For this review, take the finished solid that the model builds, in its own axes (mm). Coordinates: 2 decimals unless noted, no trailing zeros. Write each loop counter-clockwise with the first axis right and the second up, starting at its lowest first coordinate (ties: lowest second). Pieces come first, ordered by that corner, then holes. Notation, with made-up numbers: M -35.75,72.25 L 18.25,72.25 A21 cw 18.25,96.25 Z; hole C 27.25,29.25 d4. An arc over 180 degrees is marked long. One line per question, with ' | ' between items.
from build123d import *

# Parameters (mm, degrees)
CROQUIS1_R              = 9
SALIENTE_EXTRUIR1_DEPTH = 25
CROQUIS2_R              = 1.5
CORTAR_EXTRUIR1_DEPTH   = 25


with BuildPart() as part:
    # Croquis1 → Saliente-Extruir1 (new body)
    with BuildSketch(Plane.XY):
        Polygon((-22.5, 5), (-12.5, 15), (12.5, 15), (22.5, 5), (22.5, -15), (-22.5, -15), align=None)
        Circle(CROQUIS1_R, mode=Mode.SUBTRACT)
    extrude(amount=SALIENTE_EXTRUIR1_DEPTH)

    # Croquis2 → Cortar-Extruir1 (cut)
    with BuildSketch(Plane.XY.offset(25)):
        with Locations((-15, -10)):
            Circle(CROQUIS2_R)
        with Locations((15, -10)):
            Circle(CROQUIS2_R)
        with Locations((-10, 11)):
            Circle(CROQUIS2_R)
        with Locations((10, 11)):
            Circle(CROQUIS2_R)
    extrude(amount=-CORTAR_EXTRUIR1_DEPTH, mode=Mode.SUBTRACT)


solid = part.part
1) We need section D-D on y = 11. State the section outline as (x, z) points.
Responses:
outline: M -16.5,0 L -11.5,0 L -11.5,25 L -16.5,25 Z; M -8.5,0 L 8.5,0 L 8.5,25 L -8.5,25 Z; M 11.5,0 L 16.5,0 L 16.5,25 L 11.5,25 Z
2) Insertion check: pin 1 Ø11 at (x, y) = (0, 0) entering from +Z; pin 2 Ø4 at (x, y) = (-15, -10) entering from -Z. Each pin has a flat end and moves straight along its axis. Give the tip position at first contact, or say it passes through.
Responses:
pin 1: through | pin 2: z = 0
3) We need section C-C on z = 2.5. State the section outline as (x, y) points.
Responses:
outline: M -22.5,-15 L 22.5,-15 L 22.5,5 L 12.5,15 L -12.5,15 L -22.5,5 Z; hole C -15,-10 d3; hole C -10,11 d3; hole C 0,0 d18; hole C 10,11 d3; hole C 15,-10 d3
4) The part is to be moulded in two halves that separate along X. For faces 1 (the flat face through (17.4, 10.1, 12.3)), 2 (the flat face through (-17.6, 9.9, 12.3)), 3 (the flat face through (0, -10, 25)), 4 (the cylindrical face through (8.5, 11.07, 12.68)), say which applies: +X half, -X half, draft (parallel to the pull), parting line (faces both ways), or undercut.
Responses:
face 1: +X half | face 2: -X half | face 3: draft | face 4: undercut
5) To check wall thickness, follow line 1 along Y through (x, z) = (-10, 17.25); line 2 along Y through (x, z) = (15, 8); line 3 along Y through (x, z) = (-18.5, 21). State the ranges of each line that lie inside material, in increasing order. Write a range as [from, to].
Responses:
line 1: [-15, 9.5], [12.5, 15] | line 2: [-15, -11.5], [-8.5, 12.5] | line 3: [-15, 9]
6) We need section A-A on y = 0. State the section outline as (x, z) points.
Responses:
outline: M -22.5,0 L -9,0 L -9,25 L -22.5,25 Z; M 9,0 L 22.5,0 L 22.5,25 L 9,25 Z
7) We need section B-B on x = -15. State the section outline as (y, z) points.
Responses:
outline: M -15,0 L -11.5,0 L -11.5,25 L -15,25 Z; M -8.5,0 L 12.5,0 L 12.5,25 L -8.5,25 Z
